Source: three-view drawing plus pictorial views. Frame: mm from the lowest corner of the part. A direction names the side the tool comes from. Give positions to 0.01 mm unless a question says otherwise; leave off trailing zeros. Loops run counter-clockwise (first coordinate to the right, second up) from the corner with the lowest first, then second, coordinate; pieces in that order, holes last. Notation, with made-up numbers: M -2.75,37.5 L 3.25,37.5 A6 ccw 3.25,41.5 Z; hole C 63.25,1 d10. An arc over 180 degrees is marked long. Answer as a JSON object with one key per item and string values. Group by question number.
1) Section query D-D on z = 2.5. Return loops of the section in (x, y).
2) Section query B-B on x = 15. Return loops of the section in (y, z).
3) Access query for the marked faces 1, 2, 3 and 4. Directions: +Z, -Z, +X, -X, +Y, -Y. A direction counts if a zero-diameter tool reaches every point of the face in a straight line with its end or side. Return the directions, or none.
4) Section query C-C on y = 20. Return loops of the section in (x, z), plus the area to 4 significant figures.
5) Draft query along X for the marked faces 5, 6 and 7. Return one class per face: +X half, -X half, draft (parallel to the pull), parting line (faces both ways), or undercut.
6) Ray query, L1, parallel to Y at x = 15, z = 6.25; L2, parallel to X at y = 30.5, z = 9.5; L3, parallel to X at y = 23, z = 5.5. Return the intervals inside material, ascending.
7) Section query A-A on z = 7.5. Return loops of the section in (x, y).
8) First-contact query: P1, Ø3.5, axis at x = 14, z = 7, coming from the -Y side; P2, Ø4, axis at x = 14, y = 37.5, coming from the -Z side; P3, Ø0.9, axis at x = 2, y = 26.5, coming from the +Z side. Flat tips, straight axial feed; report the tip coordinate or a pass-through.
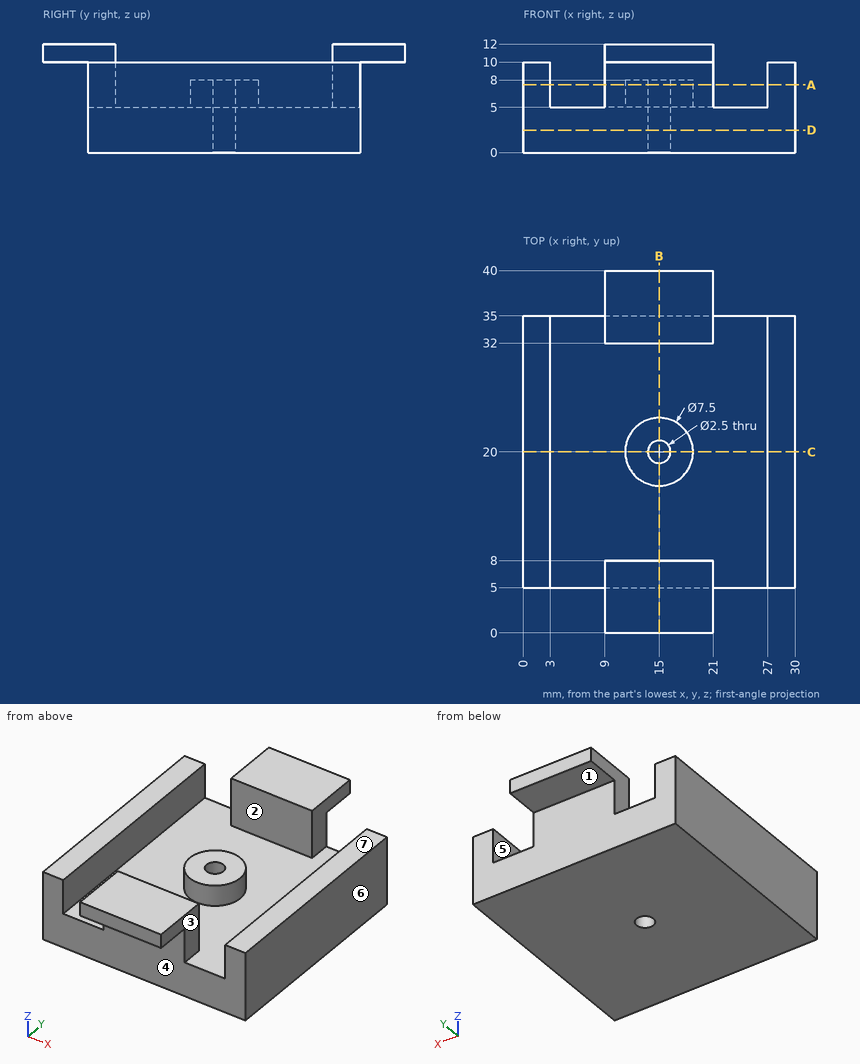
Output:
{
 "1": {"outline": "M 0,5 L 30,5 L 30,35 L 0,35 Z; hole C 15,20 d2.5"},
 "2": {"outline": "M 0,10 L 5,10 L 5,0 L 18.75,0 L 18.75,8 L 16.25,8 L 16.25,5 L 8,5 L 8,12 L 0,12 Z; M 21.25,0 L 35,0 L 35,10 L 40,10 L 40,12 L 32,12 L 32,5 L 23.75,5 L 23.75,8 L 21.25,8 Z"},
 "3": {"face 1": "-Z, +X, -X, +Y", "face 2": "+Z", "face 3": "+Z, +Y, -Y", "face 4": "-Z, +X, -X, -Y"},
 "4": {"outline": "M 0,0 L 13.75,0 L 13.75,8 L 11.25,8 L 11.25,5 L 3,5 L 3,10 L 0,10 Z; M 16.25,0 L 30,0 L 30,10 L 27,10 L 27,5 L 18.75,5 L 18.75,8 L 16.25,8 Z", "area": "182.5 mm^2"},
 "5": {"face 5": "undercut", "face 6": "+X half", "face 7": "draft"},
 "6": {"L1": "y = 5 to 8, 16.25 to 18.75, 21.25 to 23.75, 32 to 35", "L2": "x = 0 to 3, 27 to 30", "L3": "x = 0 to 3, 12.75 to 17.25, 27 to 30"},
 "7": {"outline": "M 0,5 L 3,5 L 3,35 L 0,35 Z; M 9,5 L 21,5 L 21,8 L 9,8 Z; M 9,32 L 21,32 L 21,35 L 9,35 Z; C 15,20 d7.5; M 27,5 L 30,5 L 30,35 L 27,35 Z; hole C 15,20 d2.5"},
 "8": {"P1": "stops at y = 5", "P2": "stops at z = 10", "P3": "stops at z = 10"}
}
